Source: CAD feature listing. Evaluate the final solid. Frame: model axes, mm. Face numbers are marked on the shaded views. A direction names the side the tool comes from. Coordinates: 2 decimals unless noted, no trailing zeros. Loops run counter-clockwise (first coordinate to the right, second up) from the corner with the lowest first, then second, coordinate; pieces in that order, holes last. Notation, with made-up numbers: (47, 43.5) - (73, 43.5) arc R29 cw to (73, 71.5) - close; hole circle Ø2 at (8.25, -1.5). An arc over 180 degrees is marked (long way). Use CSV: the item, a comma, the result in double quotes. Start each with the question number.
```python
from build123d import *

# Parameters (mm, degrees)
F1_DEPTH = 25
F2_R     = 5
F3_DEPTH = 25


with BuildPart() as f1:
    # F0 (on Top) → F1 (new body)
    with BuildSketch(Plane.XY):
        with BuildLine():
            Line((7.482701, 22.981227), (0, 22.981227))
            Line((0, 22.981227), (-7.482701, 22.981227))
            ThreePointArc((-7.482701, 22.981227), (-9.411064, 22.27936), (-10.437124, 20.502171))
            Line((-10.437124, 20.502171), (-14.098284, -0.261297))
            ThreePointArc((-14.098284, -0.261297), (-14.595251, -1.461082), (-15.552707, -2.338429))
            Line((-15.552707, -2.338429), (-23.001458, -6.638967))
            Line((-23.001458, -6.638967), (-22.501458, -7.504993))
            Line((-22.501458, -7.504993), (-14.648873, -2.9713))
            ThreePointArc((-14.648873, -2.9713), (-13.691417, -2.093953), (-13.19445, -0.894169))
            Line((-13.19445, -0.894169), (-9.598025, 19.502171))
            ThreePointArc((-9.598025, 19.502171), (-8.571964, 21.27936), (-6.643601, 21.981227))
            Line((-6.643601, 21.981227), (0, 21.981227))
            Line((0, 21.981227), (6.643601, 21.981227))
            ThreePointArc((6.643601, 21.981227), (8.571964, 21.27936), (9.598025, 19.502171))
            Line((9.598025, 19.502171), (13.19445, -0.894169))
            ThreePointArc((13.19445, -0.894169), (13.691417, -2.093953), (14.648873, -2.9713))
            Line((14.648873, -2.9713), (22.501458, -7.504993))
            Line((22.501458, -7.504993), (23.001458, -6.638967))
            Line((23.001458, -6.638967), (15.552707, -2.338429))
            ThreePointArc((15.552707, -2.338429), (14.595251, -1.461082), (14.098284, -0.261297))
            Line((14.098284, -0.261297), (10.437124, 20.502171))
            ThreePointArc((10.437124, 20.502171), (9.411064, 22.27936), (7.482701, 22.981227))
        make_face()
    extrude(amount=F1_DEPTH)

    # F2 (on face) → F3 (cut)
    with BuildSketch(Plane(origin=(0, 22.981227, 0), x_dir=(-1, 0, 0), z_dir=(0, 1, 0))):
        with Locations((0, 12.5)):
            Circle(F2_R)
    extrude(amount=-F3_DEPTH, mode=Mode.SUBTRACT)


solid = f1.part
```
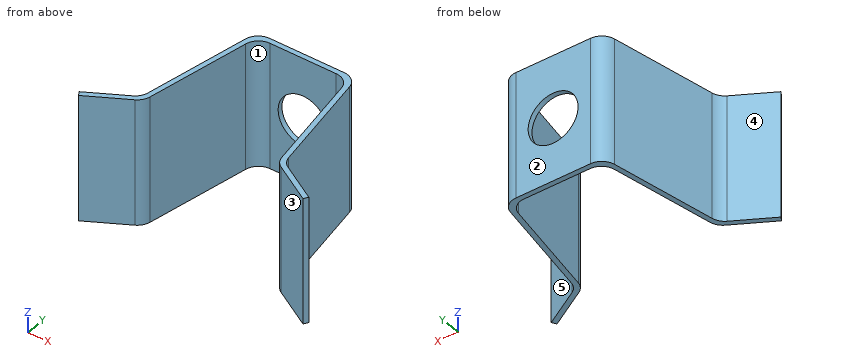
(1) Pin query (flat end, axial travel): pin 1 Ø11.5 at (x, z) = (0, 12.5) entering from +Y; pin 2 Ø4 at (y, z) = (5, 20.5) entering from -X; pin 3 Ø3 at (y, z) = (10.5, 11.5) entering from -X; pin 4 Ø1 at (y, z) = (0, 7) entering from -X. Return the tip coordinate at first contact, or that it passes through.
(2) Ray query, line 1 (Z direction, x = 0, y = 22.35); line 2 (Y direction, x = -3.5, z = 18.75); line 3 (X direction, y = 2, z = 3.25). Return the intervals inside material, ascending. Write a range as [from, to].
(3) Section C-C on y = 11. Output: boundary loops of the cut face in (x, z), plus the area to 3 significant figures.
(4) Draft query along X for the marked faces 3, 4 and 5. Return one class per face: released by +X, released by -X, zero draft, split by the parting line, or undercut.
(5) Reachability of the marked faces 1 and 2 from +Z, -Z, +X, -X, +Y, -Y: full face, straight path, thin tool, end or side. Return the list, or none.
(6) Section D-D on z = 7. Output: boundary loops of the cut face in (x, y) (3 decimals), plus the area to 3 significant figures.
(7) Section A-A on x = 0. Output: boundary loops of the cut face in (y, z).
(8) Section B-B on z = 12.5. Output: boundary loops of the cut face in (x, y) (3 decimals), plus the area to 3 significant figures.
Solution:
1,pin 1,"stops at y = 22.98"
1,pin 2,"stops at x = -13.52"
1,pin 3,"stops at x = -12.47"
1,pin 4,"stops at x = -14.15"
2,line 1,"z = [0, 7.5], [17.5, 25]"
2,line 2,"y = [21.98, 22.98]"
2,line 3,"x = [-13.7, -12.68], [12.68, 13.7]"
3,outline,"(-12.11, 0) - (-11.1, 0) - (-11.1, 25) - (-12.11, 25) - close; (11.1, 0) - (12.11, 0) - (12.11, 25) - (11.1, 25) - close"
3,area,"50.8 mm²"
4,face 3,"undercut"
4,face 4,"released by -X"
4,face 5,"released by +X"
5,face 1,"+Z, -Z, -Y"
5,face 2,"+Z, -Z, +X, -X, +Y"
6,outline,"(-23.001, -6.639) - (-22.501, -7.505) - (-14.649, -2.971) arc R3 ccw to (-13.194, -0.894) - (-9.598, 19.502) arc R3 cw to (-6.644, 21.981) - (6.644, 21.981) arc R3 cw to (9.598, 19.502) - (13.194, -0.894) arc R3 ccw to (14.649, -2.971) - (22.501, -7.505) - (23.001, -6.639) - (15.553, -2.338) arc R3 cw to (14.098, -0.261) - (10.437, 20.502) arc R3 ccw to (7.483, 22.981) - (-7.483, 22.981) arc R3 ccw to (-10.437, 20.502) - (-14.098, -0.261) arc R3 cw to (-15.553, -2.338) - close"
6,area,"89.3 mm²"
7,outline,"(21.98, 0) - (22.98, 0) - (22.98, 7.5) - (21.98, 7.5) - close; (21.98, 17.5) - (22.98, 17.5) - (22.98, 25) - (21.98, 25) - close"
8,outline,"(-23.001, -6.639) - (-22.501, -7.505) - (-14.649, -2.971) arc R3 ccw to (-13.194, -0.894) - (-9.598, 19.502) arc R3 cw to (-6.644, 21.981) - (-5, 21.981) - (-5, 22.981) - (-7.483, 22.981) arc R3 ccw to (-10.437, 20.502) - (-14.098, -0.261) arc R3 cw to (-15.553, -2.338) - close; (5, 21.981) - (6.644, 21.981) arc R3 cw to (9.598, 19.502) - (13.194, -0.894) arc R3 ccw to (14.649, -2.971) - (22.501, -7.505) - (23.001, -6.639) - (15.553, -2.338) arc R3 cw to (14.098, -0.261) - (10.437, 20.502) arc R3 ccw to (7.483, 22.981) - (5, 22.981) - close"
8,area,"79.3 mm²"
